Geometry check sheet. Reference: the model listing, model coordinates, mm. Face numbers are marked on the shaded views. A direction names the side the tool comes from. Give positions to 0.01 mm unless a question says otherwise; leave off trailing zeros. Loops run counter-clockwise (first coordinate to the right, second up) from the corner with the lowest first, then second, coordinate; pieces in that order, holes last. Notation, with made-up numbers: (80.25, 71.25) -> (120.25, 71.25) arc R16 cw to (120.25, 79.25) -> close; hole circle Ø4 at (39.5, -10). An arc over 180 degrees is marked (long way). One line per item, written item: value. Start each with the question number.
(1) Sectioned sample at B-B, the plane x = -17. Record the cut outline in (y, z), then the cut area to 3 significant figures.
(2) Sectioned sample at C-C, the plane y = 0. Record the cut outline in (x, z), then the cut area to 3 significant figures.
(3) Scan lines: line 1 along Z through (x, y) = (-12, 18.5); line 2 along Y through (x, z) = (-11.5, 119.5); line 3 along Z through (x, y) = (-3, -63.5). Record each from-to range of solid material in increasing order. Write a range as from..to.
(4) Tool access check on the marked faces 1, 2 and 3. Record the directions out of +Z, -Z, +X, -X, +Y, -Y that give a thin tool (end or side, any length) a straight path to the whole face; none if there is none.
(5) Gauge pin test, flat ends, axial feed: pin 1 Ø0.9 at (x, y) = (0.5, -66) entering from -Z; pin 2 Ø8 at (x, z) = (-15.5, 51) entering from +Y; pin 3 Ø16.5 at (x, y) = (-4, -57.5) entering from -Z. Record the tip position at first contact, or that the pin passes through.
(6) Sectioned sample at D-D, the plane z = 45.5. Record the cut outline in (x, y).
(7) Sectioned sample at A-A, the plane x = 0. Record the cut outline in (y, z), then the cut area to 3 significant figures.
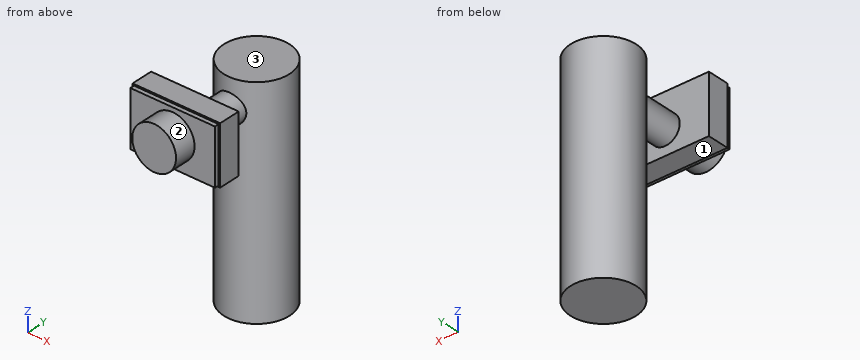
from build123d import *

# Parameters (mm, degrees)
F2_R      = 10
F3_DEPTH  = 50
F5_W      = 60
F5_H      = 40
F6_DEPTH  = 15
F0_R      = 22.5
F8_W      = 58
F8_H      = 38
F9_DEPTH  = 3
F10_R     = 15
F11_DEPTH = 15


with BuildPart() as f3:
    # F2 (on Front) → F3 (new body)
    with BuildSketch(Plane.XZ):
        with Locations((0, 130.387224)):
            Circle(F2_R)
    extrude(amount=F3_DEPTH)

    # F5 (on offset) → F6 (join)
    with BuildSketch(Plane.XZ.offset(50)):
        with Locations((0, 134.238796)):
            Rectangle(F5_W, F5_H)
    extrude(amount=F6_DEPTH)

    # F7: sweep along a path in F1
    with BuildLine(Plane.XZ) as f7_path:
        Line((0, 0), (0, 150))
    # F0 (on Top) → F7 (sweep)
    with BuildSketch(Plane.XY):
        Circle(F0_R)
    sweep(path=f7_path.line)

    # F8 (on face) → F9 (join)
    with BuildSketch(Plane.XZ.offset(65)):
        with Locations((0, 134.238796)):
            Rectangle(F8_W, F8_H)
    extrude(amount=F9_DEPTH)

    # F10 (on face) → F11 (join)
    with BuildSketch(Plane.XZ.offset(68)):
        with Locations((0, 135.238796)):
            Circle(F10_R)
    extrude(amount=F11_DEPTH)


solid = f3.part
Calculated:
1. outline: (-68, 115.24) -> (-65, 115.24) -> (-65, 114.24) -> (-50, 114.24) -> (-50, 154.24) -> (-65, 154.24) -> (-65, 153.24) -> (-68, 153.24) -> close; (-14.74, 0) -> (14.74, 0) -> (14.74, 150) -> (-14.74, 150) -> close
1. area: 5,140 mm2
2. outline: (-22.5, 0) -> (22.5, 0) -> (22.5, 150) -> (-22.5, 150) -> close
2. area: 6,750 mm2
3. line 1: z = 0..150
3. line 2: y = -68..-50, -19.34..19.34
3. line 3: z = 114.24..154.24
4. face 1: -Z, +X, -X, -Y
4. face 2: -Y
4. face 3: +Z, +X, -X, +Y
5. pin 1: stops at z = 115.24
5. pin 2: stops at y = 19.34
5. pin 3: stops at z = 114.24
6. outline: circle Ø45 at (0, 0)
7. outline: (-83, 120.24) -> (-68, 120.24) -> (-68, 115.24) -> (-65, 115.24) -> (-65, 114.24) -> (-50, 114.24) -> (-50, 120.39) -> (-22.5, 120.39) -> (-22.5, 0) -> (22.5, 0) -> (22.5, 150) -> (-22.5, 150) -> (-22.5, 140.39) -> (-50, 140.39) -> (-50, 154.24) -> (-65, 154.24) -> (-65, 153.24) -> (-68, 153.24) -> (-68, 150.24) -> (-83, 150.24) -> close
7. area: 8,460 mm2
